For this review, use the dimensioned drawing (mm, ordinates from the lowest corner) and the shaded views. Coordinates: 2 decimals unless noted, no trailing zeros. Loops run counter-clockwise (first coordinate to the right, second up) from the corner with the lowest first, then second, coordinate; pieces in that order, holes last. Notation, with made-up numbers: M 71,36 L 112,36 A22 cw 112,69 Z; hole C -21,84 d7. An arc over 180 degrees is marked long. One line per item, written item: value.
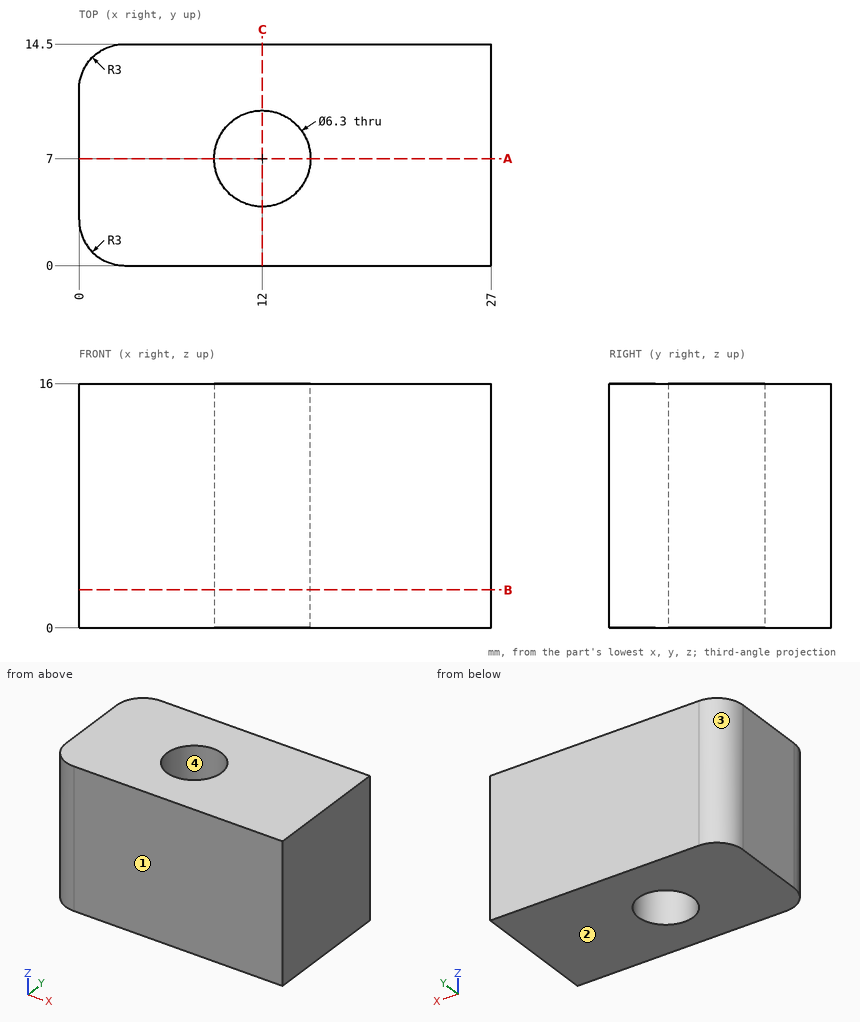
(1) Mouldability with a two-part tool opening along Y and no side actions: class the marked faces 1, 2, 3 and 4 as released by +Y, released by -Y, zero draft, split by the parting line, or undercut.
Reply:
face 1: released by -Y
face 2: zero draft
face 3: released by +Y
face 4: undercut
(2) We need section C-C on x = 12. State the section outline as (y, z) points, then the cut area to 3 significant figures.
Reply:
outline: M 0,0 L 3.85,0 L 3.85,16 L 0,16 Z; M 10.15,0 L 14.5,0 L 14.5,16 L 10.15,16 Z
area: 131 mm2
(3) To check wall thickness, follow line 1 along X through (y, z) = (7, 3.75); line 2 along Y through (x, z) = (12, 10.75); line 3 along X through (y, z) = (8, 6). State the ranges of each line that lie inside material, in increasing order. Write a range as [from, to].
Reply:
line 1: x = [0, 8.85], [15.15, 27]
line 2: y = [0, 3.85], [10.15, 14.5]
line 3: x = [0, 9.01], [14.99, 27]
(4) We need section B-B on z = 2.5. State the section outline as (x, y) points.
Reply:
outline: M 0,3 A3 ccw 3,0 L 27,0 L 27,14.5 L 3,14.5 A3 ccw 0,11.5 Z; hole C 12,7 d6.3
(5) We need section A-A on y = 7. State the section outline as (x, z) points, then the cut area to 3 significant figures.
Reply:
outline: M 0,0 L 8.85,0 L 8.85,16 L 0,16 Z; M 15.15,0 L 27,0 L 27,16 L 15.15,16 Z
area: 331 mm2
